Check sheet for the modelled part. Datum: model origin and axes. Units: mm. Round coordinates to 2 decimals unless told otherwise and drop trailing zeros. Loops run counter-clockwise (first coordinate to the right, second up) from the corner with the lowest first, then second, coordinate; pieces in that order, holes last. Notation, with made-up numbers: (54, 10) - (93, 10) arc R21 cw to (93, 37) - close; hole circle Ø5 at (72, 58). An arc over 180 degrees is marked (long way). Answer in a Markdown table with one row per item. Add a question column.
(1) Gauge pin test, flat end, axial feed: pin 1 (0.9 mm diameter, centred on y = -1.5, z = -38.5, fed in from +X). Record the tip position at first contact, or that the pin passes through.
(2) Mould release check, pull along Z, two halves, no side actions. Record for faces 1 (the flat face through (22, -2, -29.146)), 2 (the flat face through (21, -3.81, -39)), 3 (the flat face through (23.373, -2, -39)): +Z half, -Z half, draft (parallel to the pull), parting line (faces both ways), or undercut.
(3) Cross-section at B-B on y = -1.1. Enter the section's corners in (x, z).
(4) Thickness scan on line 1 along X through (y, z) = (-1.95, -47.5); line 2 along Z through (x, y) = (23.5, -3.6); line 3 along X through (y, z) = (-3, -39.75). Record the ranges inside material, lowest first.
(5) Cross-section at A-A on x = 25.5. Enter the section's corners in (y, z).
from build123d import *

# Parameters (mm, degrees)
F0_W     = 6.35
F0_H     = 8.636
F1_DEPTH = 3.81
F3_START = -0.000254
F3_DEPTH = 3.81
F4_R     = 0.2501042953
F5_DEPTH = 50.8
F6_R     = 0.381


# Not quite as in the source:
# - a feature names something its author has since deleted; it is built from what else it names


with BuildPart() as f1:
    # F0 (on Front) → F1 (new body)
    with BuildSketch(Plane.XZ):
        Polygon((27.1829397243, -29.1464989846), (17.0229397243, -29.1464989846), (17.0229397243, -34.7344989846), (23.3729397243, -34.7344989846), (27.1829397243, -34.7344989846), align=None)
        with Locations((20.1979397243, -39.0524989846)):
            Rectangle(F0_W, F0_H)
        Polygon((23.3729397243, -43.3704989846), (17.0229397243, -43.3704989846), (17.0229397243, -48.9584989846), (23.3729397243, -48.9584989846), (27.1829397243, -48.9584989846), (27.1829397243, -43.3704989846), align=None)
    extrude(amount=F1_DEPTH)

    # F2 (on face) → F3 (join)
    with BuildSketch(Plane.XZ.offset(3.81).offset(F3_START)):
        Polygon((27.1829397243, -29.1464989846), (17.0229397243, -29.1464989846), (17.0229397243, -34.7344989846), (23.3729397243, -34.7344989846), (27.1829397243, -34.7344989846), align=None)
        Polygon((27.1829397243, -43.3704989846), (23.3729397243, -43.3704989846), (17.0229397243, -43.3704989846), (17.0229397243, -48.9584989846), (27.1829397243, -48.9584989846), align=None)
    extrude(amount=-F3_DEPTH)

    # F4 (on face) → F5 (cut)
    with BuildSketch(Plane(origin=(0, 0, -48.9584989846), x_dir=(1, 0, 0), z_dir=(0, 0, -1))):
        with Locations((26.094635429, 1.904746)):
            Circle(F4_R)
        with Locations((18.1112440196, 1.904746)):
            Circle(F4_R)
    extrude(amount=-F5_DEPTH, mode=Mode.SUBTRACT)

    # F6 (call 1 of 10: OpenCascade refuses the feature's edges together)
    f6_edges = [f1.edges().sort_by_distance(p)[0] for p in [
        (27.18294, -3.81, -31.940499),
    ]]
    fillet(f6_edges, radius=F6_R)

    # F6#2 (call 2 of 10)
    f6_2_edges = [f1.edges().sort_by_distance(p)[0] for p in [
        (17.02294, -3.81, -39.052499),
    ]]
    fillet(f6_2_edges, radius=F6_R)

    # F6#3 (call 3 of 10)
    f6_3_edges = [f1.edges().sort_by_distance(p)[0] for p in [
        (27.18294, -3.81, -46.164499),
    ]]
    fillet(f6_3_edges, radius=F6_R)

    # F6#4 (call 4 of 10)
    f6_4_edges = [f1.edges().sort_by_distance(p)[0] for p in [
        (23.37294, -3.81, -39.052499),
    ]]
    fillet(f6_4_edges, radius=F6_R)

    # F6#5 (call 5 of 10)
    f6_5_edges = [f1.edges().sort_by_distance(p)[0] for p in [
        (23.37294, 0, -39.052499),
    ]]
    fillet(f6_5_edges, radius=F6_R)

    # F6#7 (call 6 of 10)
    f6_7_edges = [f1.edges().sort_by_distance(p)[0] for p in [
        (27.18294, 0.000254, -31.940499),
    ]]
    fillet(f6_7_edges, radius=F6_R)

    # F6#8 (call 7 of 10)
    f6_8_edges = [f1.edges().sort_by_distance(p)[0] for p in [
        (27.18294, 0.000254, -46.164499),
    ]]
    fillet(f6_8_edges, radius=F6_R)

    # F6#10 (call 8 of 10)
    f6_10_edges = [f1.edges().sort_by_distance(p)[0] for p in [
        (17.02294, 0, -39.052499),
    ]]
    fillet(f6_10_edges, radius=F6_R)

    # F6#6 (call 9 of 10)
    f6_6_edges = [f1.edges().sort_by_distance(p)[0] for p in [
        (17.02294, 0.000254, -31.940499),
    ]]
    fillet(f6_6_edges, radius=F6_R)

    # F6#9 (call 10 of 10)
    f6_9_edges = [f1.edges().sort_by_distance(p)[0] for p in [
        (17.02294, 0.000254, -46.164499),
    ]]
    fillet(f6_9_edges, radius=F6_R)


solid = f1.part
Answers:
| question | item | result |
|---|---|---|
| 1 | pin 1 | stops at x = 23.37 |
| 2 | face 1 | +Z half |
| 2 | face 2 | draft |
| 2 | face 3 | undercut |
| 3 | outline | (17.02, -48.96) - (27.18, -48.96) - (27.18, -43.37) - (23.37, -43.37) - (23.37, -34.73) - (27.18, -34.73) - (27.18, -29.15) - (17.02, -29.15) - close |
| 4 | line 1 | x = 17.02 to 17.87, 18.36 to 25.85, 26.34 to 27.18 |
| 4 | line 2 | z = -48.96 to -43.37, -34.73 to -29.15 |
| 4 | line 3 | x = 17.02 to 23.37 |
| 5 | outline | (-3.81, -48.96) - (0, -48.96) - (0, -43.37) - (-3.81, -43.37) - close; (-3.81, -34.73) - (0, -34.73) - (0, -29.15) - (-3.81, -29.15) - close |
